from build123d import *

# Parameters (mm, degrees)
SKETCH1_R           = 1.75
BOSS_EXTRUDE1_DEPTH = 4.5
BOSS_EXTRUDE2_DEPTH = 4.5


with BuildPart() as part:
    # Sketch1 → Boss-Extrude1 (new body)
    with BuildSketch(Plane(origin=(0, 0, 0), x_dir=(0, 0, -1), z_dir=(1, 0, 0))):
        with BuildLine():
            Line((22, 10), (5, 10))
            ThreePointArc((5, 10), (0, 5), (5, 0))
            Line((5, 0), (22, 0))
            ThreePointArc((22, 0), (27, 5), (22, 10))
        make_face()
        with Locations((5, 5)):
            Circle(SKETCH1_R, mode=Mode.SUBTRACT)
        with Locations((22, 5)):
            Circle(SKETCH1_R, mode=Mode.SUBTRACT)
    extrude(amount=BOSS_EXTRUDE1_DEPTH)

    # Sketch2 → Boss-Extrude2 (add)
    with BuildSketch(Plane(origin=(4.5, 0, 5.948752288), x_dir=(0, 0, -1), z_dir=(1, 0, 0))):
        with BuildLine():
            add(Edge.make_bspline(
                [(64.143181637, 16.951696957), (46.3659084, 27.475135201), (31.177283873, 9.75391621), (13.694974759, 10)],
                knots=[0, 0, 0, 0, 1, 1, 1, 1], degree=3))
            Line((13.694974759, 10), (26.999543269, 9.812722758))
            ThreePointArc((26.999543269, 9.812722758), (31.550747241, 5.770381866), (28.824655416, 0.327735373))
            Line((28.824655416, 0.327735373), (38.08542066, 4.824084077))
            add(Edge.make_bspline(
                [(38.08542066, 4.824084077), (45.879227883, 13.481709162), (55.04551447, 7.665553941)],
                knots=[0, 0, 0, 1, 1, 1], degree=2))
            Line((55.04551447, 7.665553941), (66.094228393, 12.348066156))
            Line((66.094228393, 12.348066156), (64.143181637, 16.951696957))
        make_face()
    extrude(amount=-BOSS_EXTRUDE2_DEPTH)


solid = part.part
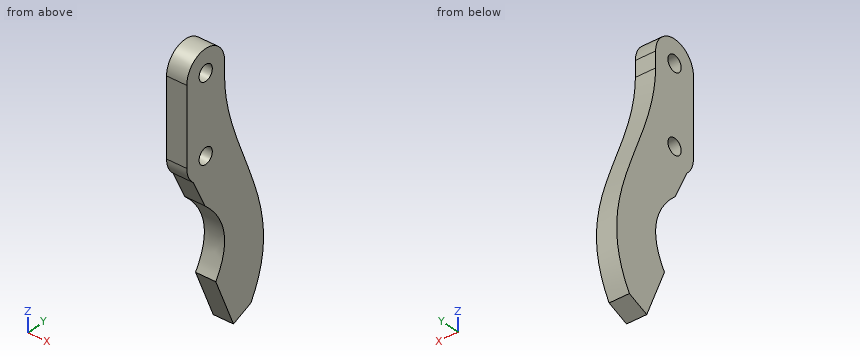
Design review of the part built by this model. Coordinates are the model's own, in mm. Give positions to 0.01 mm unless a question says otherwise; leave off trailing zeros. One line per question, with ' | ' between items. Start each with the question number.
(1) Insertion check: P1, Ø3, axis at y = 5, z = -22, coming from the -X side (1 decimal); P2, Ø1.7, axis at x = 2.5, z = -6.5, coming from the +Y side. Each pin has a flat end and moves straight along its axis. Give the tip position at first contact, or say it passes through.
(2) For line 1 (Y direction, x = 1.1, z = -5); line 2 (Z direction, x = 3.7, y = 5.25); line 3 (Y direction, x = 1.45, z = -21), list the stretches that pass through material, from the lowest coordinate up.
(3) We need section A-A (x = 3.3). State how many separate pieces and enclosed holes the cut face has, and give its area (3 significant figures).
The answers:
1) P1: passes through | P2: stops at y = 10
2) line 1: y = 0 to 3.25, 6.75 to 10 | line 2: z = -32.53 to -23.73, -20.27 to -6.73, -3.27 to -0.01 | line 3: y = 0 to 3.56, 6.44 to 12.64
3) separate pieces: 1 | enclosed holes: 2 | area: 604 mm^2
